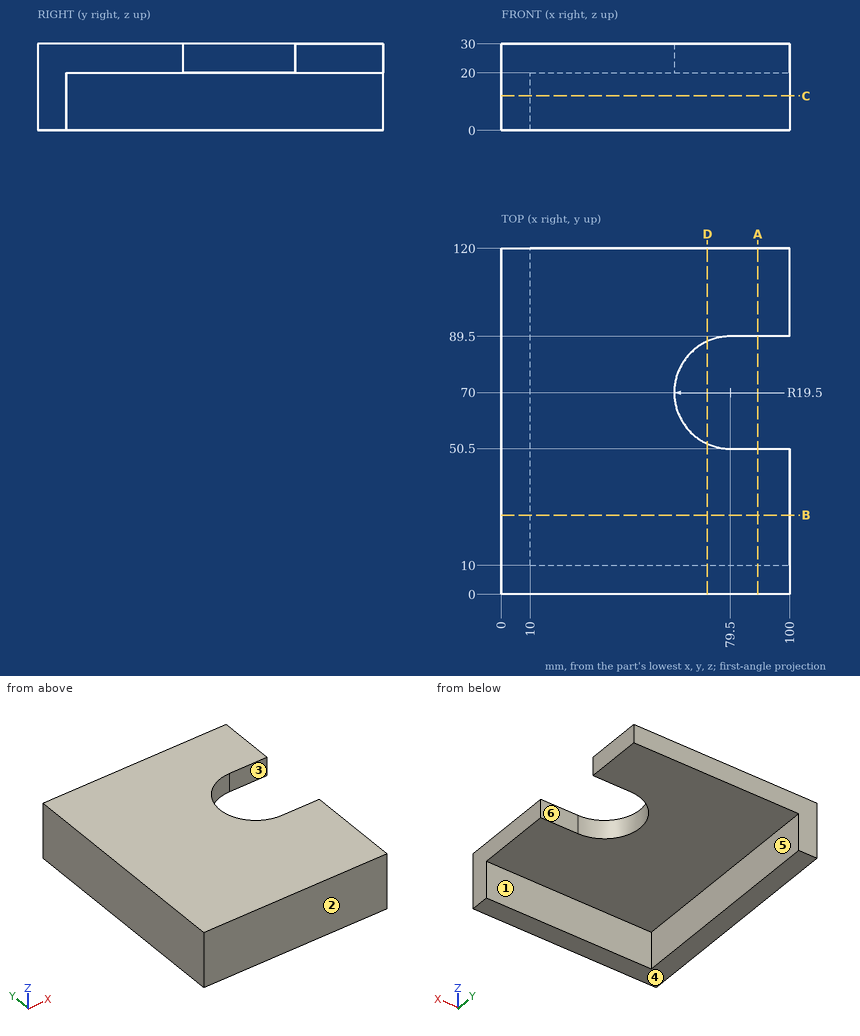
Geometry check sheet. Reference: drawing and pictorial views, mm from the part's lowest x, y, z. A direction names the side the tool comes from. Round coordinates to 2 decimals unless told otherwise and drop trailing zeros. Write each loop counter-clockwise with the first axis right and the second up, starting at its lowest first coordinate (ties: lowest second). Pieces come first, ordered by that corner, then holes.
1. Section check C-C on z = 12. Enter the section's corners in (x, y), plus the area to 3 significant figures.
2. Draft check along Y on the marked faces 1, 2 and 3. Enter one of: +Y half, -Y half, draft (parallel to the pull), parting line (faces both ways), or undercut.
3. Section check D-D on x = 71.5. Enter the section's corners in (y, z).
4. Access from +Z, -Z, +X, -X, +Y, -Y to the whole of each face (thin tool, end or side, straight path). Record for the marked faces 4, 5 and 6.
5. Scan lines: L1, parallel to Z at x = 34, y = 13; L2, parallel to Y at x = 67.5, z = 11. Record each from-to range of solid material in increasing order.
6. Gauge pin test, flat ends, axial feed: P1, Ø5, axis at x = 67.5, z = 22, coming from the -Y side; P2, Ø4, axis at x = 24.5, z = 14, coming from the +Y side; P3, Ø16, axis at y = 91.5, z = 10, coming from the +X side. Record the tip position at first contact, or that the pin passes through.
7. Section check B-B on y = 27.5. Enter the section's corners in (x, z).
8. Section check A-A on x = 89. Enter the section's corners in (y, z).
Answer:
1. outline: (0, 0) - (100, 0) - (100, 10) - (10, 10) - (10, 120) - (0, 120) - close
1. area: 2,100 mm2
2. face 1: +Y half
2. face 2: -Y half
2. face 3: undercut
3. outline: (0, 0) - (10, 0) - (10, 20) - (52.22, 20) - (52.22, 30) - (0, 30) - close; (87.78, 20) - (120, 20) - (120, 30) - (87.78, 30) - close
4. face 4: -Z, +X, -X, +Y, -Y
4. face 5: -Z, +X, +Y
4. face 6: +Z, -Z, +X
5. L1: z = 20 to 30
5. L2: y = 0 to 10
6. P1: stops at y = 0
6. P2: stops at y = 10
6. P3: stops at x = 10
7. outline: (0, 0) - (10, 0) - (10, 20) - (100, 20) - (100, 30) - (0, 30) - close
8. outline: (0, 0) - (10, 0) - (10, 20) - (50.5, 20) - (50.5, 30) - (0, 30) - close; (89.5, 20) - (120, 20) - (120, 30) - (89.5, 30) - close
